```python
from build123d import *

# Parameters (mm, degrees)
F0_W     = 22
F0_H     = 30
F0_R     = 4
F0_R_2   = 1.5
F0_H_2   = 7.1
F0_H_3   = 125.8
F0_R_3   = 1.8
F1_DEPTH = 10
F2_DEPTH = 4.5
F3_DEPTH = 17
F4_DEPTH = 13.2
F5_R     = 1.5
F6_DEPTH = 15
F7_R     = 1.5
F8_DEPTH = 15
F9_DEPTH = 2


# Not quite as in the source:
# - a feature names something its author has since deleted; it is built from what else it names


with BuildPart() as f1:
    # F0 (on Top) → F1 (new body)
    with BuildSketch(Plane.XY):
        with Locations((29, -85)):
            Rectangle(F0_W, F0_H)
        with BuildLine():
            Line((-40, -100), (18, -100))
            Line((18, -100), (18, -70))
            Line((18, -70), (18, -62.9))
            Line((18, -62.9), (18, 62.9))
            Line((18, 62.9), (18, 70))
            Line((18, 70), (18, 100))
            Line((18, 100), (-40, 100))
            Line((-40, 100), (-40, 38.55))
            Line((-40, 38.55), (-10.3232520311, 38.55))
            Line((-10.3232520311, 38.55), (-10.3232520311, 37.75))
            Line((-10.3232520311, 37.75), (-2.3232520311, 37.75))
            ThreePointArc((-2.3232520311, 37.75), (3.6, 35), (-2.3232520311, 32.25))
            Line((-2.3232520311, 32.25), (-10.3232520311, 32.25))
            Line((-10.3232520311, 32.25), (-10.3232520311, 31.45))
            Line((-10.3232520311, 31.45), (-40, 31.45))
            Line((-40, 31.45), (-40, 18.55))
            Line((-40, 18.55), (-10.3232520311, 18.55))
            Line((-10.3232520311, 18.55), (-10.3232520311, 17.75))
            Line((-10.3232520311, 17.75), (-2.3232520311, 17.75))
            ThreePointArc((-2.3232520311, 17.75), (3.6, 15), (-2.3232520311, 12.25))
            Line((-2.3232520311, 12.25), (-10.3232520311, 12.25))
            Line((-10.3232520311, 12.25), (-10.3232520311, 11.45))
            Line((-10.3232520311, 11.45), (-40, 11.45))
            Line((-40, 11.45), (-40, -11.45))
            Line((-40, -11.45), (-10.3232520311, -11.45))
            Line((-10.3232520311, -11.45), (-10.3232520311, -12.25))
            Line((-10.3232520311, -12.25), (-2.3232520311, -12.25))
            ThreePointArc((-2.3232520311, -12.25), (3.6, -15), (-2.3232520311, -17.75))
            Line((-2.3232520311, -17.75), (-10.3232520311, -17.75))
            Line((-10.3232520311, -17.75), (-10.3232520311, -18.55))
            Line((-10.3232520311, -18.55), (-40, -18.55))
            Line((-40, -18.55), (-40, -31.45))
            Line((-40, -31.45), (-10.3232520311, -31.45))
            Line((-10.3232520311, -31.45), (-10.3232520311, -32.25))
            Line((-10.3232520311, -32.25), (-2.3232520311, -32.25))
            ThreePointArc((-2.3232520311, -32.25), (3.6, -35), (-2.3232520311, -37.75))
            Line((-2.3232520311, -37.75), (-10.3232520311, -37.75))
            Line((-10.3232520311, -37.75), (-10.3232520311, -38.55))
            Line((-10.3232520311, -38.55), (-40, -38.55))
            Line((-40, -38.55), (-40, -100))
        make_face()
        with Locations((0, -88)):
            Circle(F0_R, mode=Mode.SUBTRACT)
        with Locations((0, -66.45)):
            Circle(F0_R_2, mode=Mode.SUBTRACT)
        with Locations((0, 66.45)):
            Circle(F0_R_2, mode=Mode.SUBTRACT)
        with Locations((0, 88)):
            Circle(F0_R, mode=Mode.SUBTRACT)
        with Locations((29, -66.45)):
            Rectangle(F0_W, F0_H_2)
        with Locations((29, 0)):
            Rectangle(F0_W, F0_H_3)
        Polygon((-40, -31.45), (-40, -38.55), (-10.3232520311, -38.55), (-10.3232520311, -37.75), (-10.3232520311, -32.25), (-10.3232520311, -31.45), align=None)
        with Locations((29, 66.45)):
            Rectangle(F0_W, F0_H_2)
        with Locations((29, 85)):
            Rectangle(F0_W, F0_H)
        Polygon((-40, -11.45), (-40, -18.55), (-10.3232520311, -18.55), (-10.3232520311, -17.75), (-10.3232520311, -12.25), (-10.3232520311, -11.45), align=None)
        Polygon((-40, 18.55), (-40, 11.45), (-10.3232520311, 11.45), (-10.3232520311, 12.25), (-10.3232520311, 17.75), (-10.3232520311, 18.55), align=None)
        Polygon((-10.3232520311, 38.55), (-40, 38.55), (-40, 31.45), (-10.3232520311, 31.45), (-10.3232520311, 32.25), (-10.3232520311, 37.75), align=None)
        with BuildLine():
            Line((-10.3232520311, 17.75), (-10.3232520311, 12.25))
            Line((-10.3232520311, 12.25), (-2.3232520311, 12.25))
            ThreePointArc((-2.3232520311, 12.25), (3.6, 15), (-2.3232520311, 17.75))
            Line((-2.3232520311, 17.75), (-10.3232520311, 17.75))
        make_face()
        with Locations((0, 15)):
            Circle(F0_R_3, mode=Mode.SUBTRACT)
        with BuildLine():
            Line((-2.3232520311, 37.75), (-10.3232520311, 37.75))
            Line((-10.3232520311, 37.75), (-10.3232520311, 32.25))
            Line((-10.3232520311, 32.25), (-2.3232520311, 32.25))
            ThreePointArc((-2.3232520311, 32.25), (3.6, 35), (-2.3232520311, 37.75))
        make_face()
        with Locations((0, 35)):
            Circle(F0_R_3, mode=Mode.SUBTRACT)
        with BuildLine():
            Line((-10.3232520311, -12.25), (-10.3232520311, -17.75))
            Line((-10.3232520311, -17.75), (-2.3232520311, -17.75))
            ThreePointArc((-2.3232520311, -17.75), (3.6, -15), (-2.3232520311, -12.25))
            Line((-2.3232520311, -12.25), (-10.3232520311, -12.25))
        make_face()
        with Locations((0, -15)):
            Circle(F0_R_3, mode=Mode.SUBTRACT)
        with BuildLine():
            Line((-10.3232520311, -32.25), (-10.3232520311, -37.75))
            Line((-10.3232520311, -37.75), (-2.3232520311, -37.75))
            ThreePointArc((-2.3232520311, -37.75), (3.6, -35), (-2.3232520311, -32.25))
            Line((-2.3232520311, -32.25), (-10.3232520311, -32.25))
        make_face()
        with Locations((0, -35)):
            Circle(F0_R_3, mode=Mode.SUBTRACT)
    extrude(amount=-F1_DEPTH)

    # F0 (on Top) → F2 (cut)
    with BuildSketch(Plane.XY):
        with BuildLine():
            Line((-10.3232520311, -32.25), (-10.3232520311, -37.75))
            Line((-10.3232520311, -37.75), (-2.3232520311, -37.75))
            ThreePointArc((-2.3232520311, -37.75), (3.6, -35), (-2.3232520311, -32.25))
            Line((-2.3232520311, -32.25), (-10.3232520311, -32.25))
        make_face()
        with Locations((0, -35)):
            Circle(F0_R_3, mode=Mode.SUBTRACT)
        with BuildLine():
            Line((-10.3232520311, -12.25), (-10.3232520311, -17.75))
            Line((-10.3232520311, -17.75), (-2.3232520311, -17.75))
            ThreePointArc((-2.3232520311, -17.75), (3.6, -15), (-2.3232520311, -12.25))
            Line((-2.3232520311, -12.25), (-10.3232520311, -12.25))
        make_face()
        with Locations((0, -15)):
            Circle(F0_R_3, mode=Mode.SUBTRACT)
        with BuildLine():
            Line((-10.3232520311, 17.75), (-10.3232520311, 12.25))
            Line((-10.3232520311, 12.25), (-2.3232520311, 12.25))
            ThreePointArc((-2.3232520311, 12.25), (3.6, 15), (-2.3232520311, 17.75))
            Line((-2.3232520311, 17.75), (-10.3232520311, 17.75))
        make_face()
        with Locations((0, 15)):
            Circle(F0_R_3, mode=Mode.SUBTRACT)
        with BuildLine():
            Line((-2.3232520311, 37.75), (-10.3232520311, 37.75))
            Line((-10.3232520311, 37.75), (-10.3232520311, 32.25))
            Line((-10.3232520311, 32.25), (-2.3232520311, 32.25))
            ThreePointArc((-2.3232520311, 32.25), (3.6, 35), (-2.3232520311, 37.75))
        make_face()
        with Locations((0, 35)):
            Circle(F0_R_3, mode=Mode.SUBTRACT)
    extrude(amount=-F2_DEPTH, mode=Mode.SUBTRACT)

    # F0 (on Top) → F3 (join)
    with BuildSketch(Plane.XY):
        with Locations((29, -85)):
            Rectangle(F0_W, F0_H)
        with Locations((29, 85)):
            Rectangle(F0_W, F0_H)
        with Locations((29, 0)):
            Rectangle(F0_W, F0_H_3)
    extrude(amount=F3_DEPTH)

    # F0 (on Top) → F4 (join)
    with BuildSketch(Plane.XY):
        with Locations((29, 66.45)):
            Rectangle(F0_W, F0_H_2)
        with Locations((29, -66.45)):
            Rectangle(F0_W, F0_H_2)
    extrude(amount=F4_DEPTH)

    # F5 (on face) → F6 (cut)
    with BuildSketch(Plane(origin=(0, 100, 0), x_dir=(-1, 0, 0), z_dir=(0, 1, 0))):
        with Locations((0, -5)):
            Circle(F5_R)
    extrude(amount=-F6_DEPTH, mode=Mode.SUBTRACT)

    # F7 (on face) → F8 (cut)
    with BuildSketch(Plane.XZ.offset(100)):
        with Locations((0, -5)):
            Circle(F7_R)
    extrude(amount=-F8_DEPTH, mode=Mode.SUBTRACT)

    # F0 (on Top) → F9 (cut)
    with BuildSketch(Plane.XY):
        Polygon((-10.3232520311, 38.55), (-40, 38.55), (-40, 31.45), (-10.3232520311, 31.45), (-10.3232520311, 32.25), (-10.3232520311, 37.75), align=None)
        Polygon((-40, 18.55), (-40, 11.45), (-10.3232520311, 11.45), (-10.3232520311, 12.25), (-10.3232520311, 17.75), (-10.3232520311, 18.55), align=None)
        Polygon((-40, -11.45), (-40, -18.55), (-10.3232520311, -18.55), (-10.3232520311, -17.75), (-10.3232520311, -12.25), (-10.3232520311, -11.45), align=None)
        Polygon((-40, -31.45), (-40, -38.55), (-10.3232520311, -38.55), (-10.3232520311, -37.75), (-10.3232520311, -32.25), (-10.3232520311, -31.45), align=None)
    extrude(amount=-F9_DEPTH, mode=Mode.SUBTRACT)


solid = f1.part
```
Input: part model. Units: mm. Frame: model coordinates. A direction names the side the tool comes from. Coordinates: 2 decimals unless noted, no trailing zeros. Write each loop counter-clockwise with the first axis right and the second up, starting at its lowest first coordinate (ties: lowest second). Pieces come first, ordered by that corner, then holes. Notation, with made-up numbers: (-34.5, -29) - (21.5, -29) arc R26 cw to (21.5, -14) - close; hole circle Ø4 at (71.5, 75). An arc over 180 degrees is marked (long way). Put each result on its own line as item: value. Start each with the question number.
1) Cut plane D-D (y = 79.5). Return the cut outline in (x, z).
2) Reachability of faces 4 (the face through (29, 85, 17)), 5 (the face through (3.6, -15.1, -2.2)), 6 (the face through (29, 66, 13.2)) from +Z, -Z, +X, -X, +Y, -Y: full face, straight path, thin tool, end or side. Return the list, or none.
3) Contact query for flat-ended pins moving along their axis: pin 1 (6 mm diameter, centred on y = 54, z = 4, fed in from -X); pin 2 (6 mm diameter, centred on y = -64.5, z = 2.5, fed in from -X); pin 3 (0.6 mm diameter, centred on y = -38, z = -1.5, fed in from -X); pin 4 (2.5 mm diameter, centred on x = 0, z = -5, fed in from -Y). Output: stop coordinate, or through.
4) Cut plane B-B (z = 15). Return the cut outline in (x, y).
5) Mould query, pull axis X, two halves, no side actions, for faces 1 (the face through (-0.234, 36.785, -7.212)), 2 (the face through (40, -1, 3)), 3 (the face through (-25, 35, -2)). Classes: pulls with the +X half, pulls with the -X half, needs draft (parallel to the pull), parting line crosses it, or undercut.
6) Cut plane A-A (y = -88). Return the cut outline in (x, z), plus the area to 3 significant figures.
7) Cut plane C-C (x = -32.5). Return the cut outline in (y, z), plus the area to 3 significant figures.
8) Ray query, L1, parallel to Z at x = 0, y = -94.5; L2, parallel to X at y = -94, z = -5; L3, parallel to X at y = 81.5, z = 1.75. Return the intervals inside material, ascending.
Resolved:
1. outline: (-40, -10) - (40, -10) - (40, 17) - (18, 17) - (18, 0) - (-40, 0) - close
2. face 4: +Z, +X, -X, +Y, -Y
2. face 5: +Z
2. face 6: +Z, +X, -X
3. pin 1: stops at x = 18
3. pin 2: stops at x = -40
3. pin 3: stops at x = -10.32
3. pin 4: stops at y = -84.2
4. outline: (18, -100) - (40, -100) - (40, -70) - (18, -70) - close; (18, -62.9) - (40, -62.9) - (40, 62.9) - (18, 62.9) - close; (18, 70) - (40, 70) - (40, 100) - (18, 100) - close
5. face 1: undercut
5. face 2: pulls with the +X half
5. face 3: needs draft
6. outline: (-40, -10) - (-4, -10) - (-4, 0) - (-40, 0) - close; (4, -10) - (40, -10) - (40, 17) - (18, 17) - (18, 0) - (4, 0) - close
6. area: 1,090 mm2
7. outline: (-100, -10) - (100, -10) - (100, 0) - (38.55, 0) - (38.55, -2) - (31.45, -2) - (31.45, 0) - (18.55, 0) - (18.55, -2) - (11.45, -2) - (11.45, 0) - (-11.45, 0) - (-11.45, -2) - (-18.55, -2) - (-18.55, 0) - (-31.45, 0) - (-31.45, -2) - (-38.55, -2) - (-38.55, 0) - (-100, 0) - close
7. area: 1,940 mm2
8. L1: z = -10 to -6.5, -3.5 to 0
8. L2: x = -40 to -1.5, 1.5 to 40
8. L3: x = 18 to 40
